For this review, use the dimensioned drawing (mm, ordinates from the lowest corner) and the shaded views. Coordinates: 2 decimals unless noted, no trailing zeros. Write each loop counter-clockwise with the first axis right and the second up, starting at its lowest first coordinate (ties: lowest second). Pieces come first, ordered by that corner, then holes. Notation, with made-up numbers: (27, 53) -> (69, 53) arc R5 ccw to (69, 62) -> close; hole circle Ø7 at (8.25, 81). An arc over 180 degrees is marked (long way). Return JSON: item names as keys, results as strings. Group by question number.
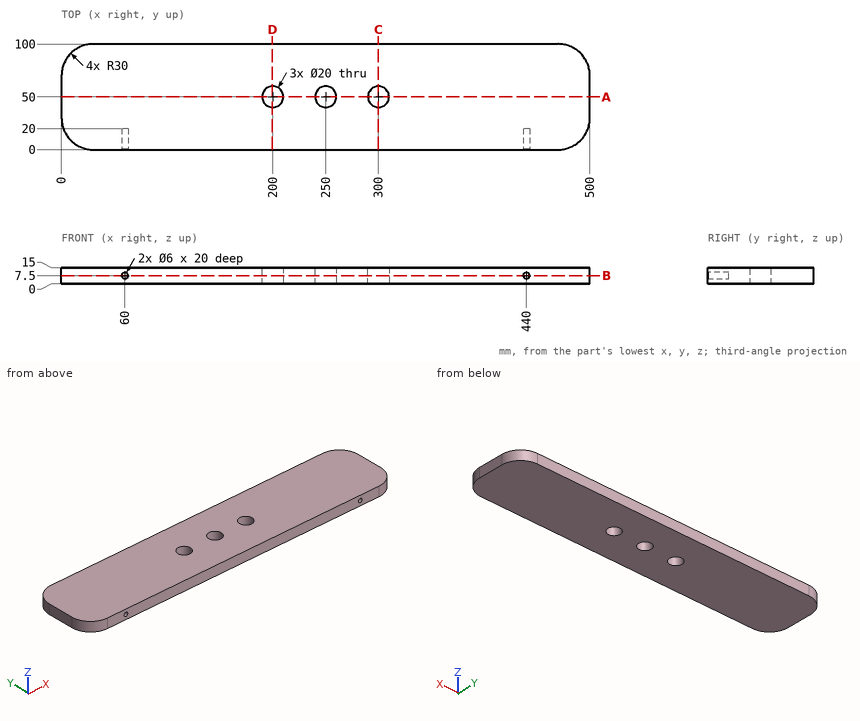
Q1. For P1, Ø2, axis at y = 23, z = 5, coming from the -X side; P2, Ø8, axis at y = 15, z = 5.5, coming from the -X side; P3, Ø3, axis at y = 74.5, z = 12, coming from the +X side, all flat-tipped, find the tip position at first contact; note any pin that passes through.
Q2. We need section C-C on x = 300. Write out the cut boundary in (y, z), plus the area to 3 significant figures.
Q3. We need section D-D on x = 199.5. Write out the cut boundary in (y, z).
Q4. We need section A-A on y = 50. Write out the cut boundary in (x, z).
Q5. We need section B-B on z = 7.5. Write out the cut boundary in (x, y), plus the area to 3 significant figures.
Q6. Wall thickness on L1, parallel to X at y = 14, z = 7.75; L2, parallel to X at y = 8.5, z = 7.5; L3, parallel to X at y = 49.5, z = 6.5: over which ranges is each line inside the solid? List them lowest first.
Findings below:
{
 "1": {"P1": "stops at x = 0.61", "P2": "stops at x = 2.09", "P3": "stops at x = 499.85"},
 "2": {"outline": "(0, 0) -> (40, 0) -> (40, 15) -> (0, 15) -> close; (60, 0) -> (100, 0) -> (100, 15) -> (60, 15) -> close", "area": "1,200 mm^2"},
 "3": {"outline": "(0, 0) -> (40.01, 0) -> (40.01, 15) -> (0, 15) -> close; (59.99, 0) -> (100, 0) -> (100, 15) -> (59.99, 15) -> close"},
 "4": {"outline": "(0, 0) -> (190, 0) -> (190, 15) -> (0, 15) -> close; (210, 0) -> (240, 0) -> (240, 15) -> (210, 15) -> close; (260, 0) -> (290, 0) -> (290, 15) -> (260, 15) -> close; (310, 0) -> (500, 0) -> (500, 15) -> (310, 15) -> close"},
 "5": {"outline": "(0, 30) arc R30 ccw to (30, 0) -> (57, 0) -> (57, 20) -> (63, 20) -> (63, 0) -> (437, 0) -> (437, 20) -> (443, 20) -> (443, 0) -> (470, 0) arc R30 ccw to (500, 30) -> (500, 70) arc R30 ccw to (470, 100) -> (30, 100) arc R30 ccw to (0, 70) -> close; hole circle Ø20 at (200, 50); hole circle Ø20 at (250, 50); hole circle Ø20 at (300, 50)", "area": "48,000 mm^2"},
 "6": {"L1": "x = 4.62 to 57.01, 62.99 to 437.01, 442.99 to 495.38", "L2": "x = 9.08 to 57, 63 to 437, 443 to 490.92", "L3": "x = 0 to 190.01, 209.99 to 240.01, 259.99 to 290.01, 309.99 to 500"}
}
